from build123d import *

# Parameters (mm, degrees)
SKETCH_1_W              = 56
SKETCH_1_H              = 48
EXTRUDE_1_DEPTH         = 10
SKETCH_2_R              = 11
CUT_EXTRUDE_1_DEPTH     = 10
HOLE_WIZARD_3_5_3_5_1_D = 3.5
SKETCH_8_W              = 56
SKETCH_8_H              = 10
EXTRUDE_2_DEPTH         = 12
HOLE_WIZARD_5_5_5_5_1_D = 5.5
SKETCH_11_R             = 3
CUT_EXTRUDE_2_DEPTH     = 16
SKETCH_13_R             = 3
CUT_EXTRUDE_3_DEPTH     = 4
CHAMFER_1_SIZE          = 1
CHAMFER_2_SIZE          = 1


with BuildPart() as part:
    # 草图1 → 凸台-拉伸1 (new body)
    with BuildSketch(Plane(origin=(0, 0, 0), x_dir=(1, 0, 0), z_dir=(0, 1, 0))):
        with Locations((28, 24)):
            Rectangle(SKETCH_1_W, SKETCH_1_H)
    extrude(amount=EXTRUDE_1_DEPTH)

    # 草图2 → 切除-拉伸1 (cut)
    with BuildSketch(Plane(origin=(0, 10, 0), x_dir=(1, 0, 0), z_dir=(0, 1, 0))):
        with Locations(Location((28, 25, 0), (0, 0, 270))):
            Circle(SKETCH_2_R)
    extrude(amount=-CUT_EXTRUDE_1_DEPTH, mode=Mode.SUBTRACT)

    # Ø3.5 (3.5) 直径孔1 (through all)
    with Locations(Plane(origin=(0, 10, 0), x_dir=(1, 0, 0), z_dir=(0, 1, 0))):
        with Locations((12.5, 40.5), (43.5, 40.5), (43.5, 9.5), (12.5, 9.5)):
            Hole(HOLE_WIZARD_3_5_3_5_1_D / 2)

    # 草图8 → 凸台-拉伸2 (add)
    with BuildSketch(Plane(origin=(0, 10, 0), x_dir=(1, 0, 0), z_dir=(0, 1, 0))):
        with Locations((28, 5)):
            Rectangle(SKETCH_8_W, SKETCH_8_H)
    extrude(amount=EXTRUDE_2_DEPTH)

    # Ø5.5 (5.5) 直径孔1 (through all)
    with Locations(Plane(origin=(0, 0, -10), x_dir=(-1, 0, 0), z_dir=(0, 0, -1))):
        with Locations((-51, 16), (-5, 16)):
            Hole(HOLE_WIZARD_5_5_5_5_1_D / 2)

    # 草图11 → 切除-拉伸2 (cut)
    with BuildSketch(Plane(origin=(0, 22, 0), x_dir=(1, 0, 0), z_dir=(0, 1, 0))):
        with Locations(Location((12.5, 9.5, 0), (0, 0, 270))):
            Circle(SKETCH_11_R)
        with Locations(Location((43.5, 9.5, 0), (0, 0, 270))):
            Circle(SKETCH_11_R)
    extrude(amount=-CUT_EXTRUDE_2_DEPTH, mode=Mode.SUBTRACT)

    # 草图13 → 切除-拉伸3 (cut)
    with BuildSketch(Plane(origin=(0, 10, 0), x_dir=(1, 0, 0), z_dir=(0, 1, 0))):
        with Locations(Location((12.5, 40.5, 0), (0, 0, 270))):
            Circle(SKETCH_13_R)
        with Locations(Location((43.5, 40.5, 0), (0, 0, 270))):
            Circle(SKETCH_13_R)
    extrude(amount=-CUT_EXTRUDE_3_DEPTH, mode=Mode.SUBTRACT)

    # 倒角1
    chamfer_1_edges = [part.edges().sort_by_distance(p)[0] for p in [
        (56, 5, -48),
        (0, 5, -48),
    ]]
    chamfer(chamfer_1_edges, length=CHAMFER_1_SIZE)

    # 倒角2
    chamfer_2_edges = [part.edges().sort_by_distance(p)[0] for p in [
        (56, 22, -5),
        (0, 22, -5),
    ]]
    chamfer(chamfer_2_edges, length=CHAMFER_2_SIZE)


solid = part.part
The listing builds one solid part. Answer for the finished solid, in the listing's coordinates (mm). A direction names the side the tool comes from. Coordinates: 2 decimals unless noted, no trailing zeros. Loops run counter-clockwise (first coordinate to the right, second up) from the corner with the lowest first, then second, coordinate; pieces in that order, holes last.
1) Find the intervals of material crossed by L1, parallel to X at y = 7.5, z = -41; L2, parallel to Z at x = 12.5, y = 3.05; L3, parallel to X at y = 3.75, z = -40.5, in increasing order.
2) Find section A-A on x = 28. Write down the section's boundary in (y, z), then the cut area to 3 significant figures.
3) Find section B-B on y = 16. Write down the section's boundary in (x, z).
4) Flat-ended cylindrical pins translate along their axes: pin 1 Ø4.5 at (x, z) = (43.5, -40.5) entering from -Y; pin 2 Ø1.5 at (x, z) = (41.5, -21) entering from +Y; pin 3 Ø3 at (x, z) = (11.5, -41) entering from +Y; pin 4 Ø6 at (x, y) = (30, 18.5) entering from -Z. Find the tip coordinate at first contact, or state that the pin passes through.
5) Find section D-D on z = -40.5. Write down the section's boundary in (x, y), then the cut area to 3 significant figures.
6) A tool of negligible diameter and unlimited length cuts with its end or side. For faces 4 (the face through (51, 13, -10)), 5 (the face through (11.6, 3, -11)), 6 (the face through (42, 6, -8)), from which of +Z, -Z, +X, -X, +Y, -Y can it reach the whole face along a straight path? Write none if from no direction.
7) Determine the mould class of faces 1 (the face through (5, 13, -10)), 2 (the face through (4.642, 18.727, -4.93)), 3 (the face through (11, 6, -39)) for opening direction Y: pulls with the +Y half, pulls with the -Y half, needs draft (parallel to the pull), parting line crosses it, or undercut.
8) Find section C-C on z = -25. Write down the section's boundary in (x, y).
Values:
1. L1: x = 0 to 9.54, 15.46 to 40.54, 46.46 to 56
1. L2: z = -48 to -42.25, -38.75 to -11.25, -7.75 to 0
1. L3: x = 0 to 10.75, 14.25 to 41.75, 45.25 to 56
2. outline: (0, -48) - (10, -48) - (10, -36) - (0, -36) - close; (0, -14) - (10, -14) - (10, -10) - (22, -10) - (22, 0) - (0, 0) - close
2. area: 380 mm2
3. outline: (0, -10) - (2.25, -10) - (2.25, 0) - (0, 0) - close; (7.75, -10) - (9.54, -10) arc R3 cw (long way) to (15.46, -10) - (40.54, -10) arc R3 cw (long way) to (46.46, -10) - (48.25, -10) - (48.25, 0) - (7.75, 0) - close; (53.75, -10) - (56, -10) - (56, 0) - (53.75, 0) - close
4. pin 1: stops at y = 0
4. pin 2: stops at y = 10
4. pin 3: stops at y = 6
4. pin 4: stops at z = -10
5. outline: (0, 0) - (10.75, 0) - (10.75, 6) - (9.5, 6) - (9.5, 10) - (0, 10) - close; (14.25, 0) - (41.75, 0) - (41.75, 6) - (40.5, 6) - (40.5, 10) - (15.5, 10) - (15.5, 6) - (14.25, 6) - close; (45.25, 0) - (56, 0) - (56, 10) - (46.5, 10) - (46.5, 6) - (45.25, 6) - close
5. area: 470 mm2
6. face 4: -Z, +X, -X, +Y
6. face 5: +Y, -Y
6. face 6: +Y
7. face 1: needs draft
7. face 2: undercut
7. face 3: pulls with the +Y half
8. outline: (0, 0) - (17, 0) - (17, 10) - (0, 10) - close; (39, 0) - (56, 0) - (56, 10) - (39, 10) - close
